Geometry: final body of the model. Coordinates: model frame, mm. A direction names the side the tool comes from. Give positions to 0.01 mm unless a question says otherwise; leave off trailing zeros. Write each loop counter-clockwise with the first axis right and the second up, starting at its lowest first coordinate (ties: lowest second). Pieces come first, ordered by that corner, then holes.
Q1. Line query: line 1 (Y direction, x = 32.35, z = 12.75); line 2 (Y direction, x = 38.5, z = 16.75); line 3 (Y direction, x = -44, z = 17). Output: solid intervals per line, ascending.
Q2. Pin query (flat end, axial travel): pin 1 Ø2 at (x, y) = (-25, 35) entering from -Z; pin 2 Ø2 at (x, y) = (-32.35, 35) entering from +Z; pin 3 Ø6 at (y, z) = (11.5, 6) entering from -X. Return the tip coordinate at first contact, or that it passes through.
Q3. Section A-A (z = 14.5). State how many separate pieces and enclosed holes the cut face has, plus the area to 3 significant figures.
Q4. Mould query, pull axis X, two halves, no side actions, for faces 1 (the cylindrical face through (-41.86, 31.1, 1.97)), 2 (the flat face through (41, 35, 19.5)), 3 (the flat face through (-33, 33, 17.5)). Classes: +X half, -X half, draft (parallel to the pull), parting line (faces both ways), or undercut.
Q5. Reachability of faces 4 (the flat face through (0, -38, 2)), 5 (the flat face through (44.05, 35, 11)), 6 (the flat face through (20.7, -44, 2)) from +Z, -Z, +X, -X, +Y, -Y: full face, straight path, thin tool, end or side. Return the list, or none.
Q6. Section B-B (y = -22.5). Return the cut outline in (x, z).
from build123d import *

# Parameters (mm, degrees)
SKETCH_R        = 1
SKETCH_W        = 23.3
SKETCH_H        = 12.8
SKETCH_W_2      = 76
SKETCH_H_2      = 21
SKETCH_W_3      = 24
SKETCH_H_3      = 16
PAD_DEPTH       = 4
SKETCH005_R     = 1.25
POCKET001_DEPTH = 5
SKETCH002_W     = 23.4
SKETCH002_H     = 6
SKETCH002_W_2   = 3
SKETCH002_H_2   = 30
PAD001_DEPTH    = 13.5
SKETCH008_R     = 1.4
POCKET_DEPTH    = 11
SKETCH007_R     = 1.25
PAD002_DEPTH    = 2
SKETCH004_W     = 19
SKETCH004_H     = 12
POCKET002_DEPTH = 5
SKETCH009_R     = 1.25
POCKET003_DEPTH = 11


with BuildPart() as part:
    # Sketch → Pad (new body)
    with BuildSketch(Plane.XY):
        with BuildLine():
            Line((-11.7, 38), (11.7, 38))
            ThreePointArc((11.7, 38), (13.82132, 38.87868), (14.7, 41))
            Line((14.7, 41), (14.7, 50.8))
            ThreePointArc((17.7, 53.8), (15.57868, 52.92132), (14.7, 50.8))
            Line((17.7, 53.8), (47, 53.8))
            ThreePointArc((50, 50.8), (49.12132, 52.92132), (47, 53.8))
            Line((50, 50.8), (50, 35))
            ThreePointArc((47, 32), (49.12132, 32.87868), (50, 35))
            Line((47, 32), (44, 32))
            ThreePointArc((44, 32), (41.87868, 31.12132), (41, 29))
            Line((41, 29), (41, -29))
            ThreePointArc((41, -29), (41.87868, -31.12132), (44, -32))
            Line((44, -32), (47, -32))
            ThreePointArc((50, -35), (49.12132, -32.87868), (47, -32))
            Line((50, -35), (50, -50.8))
            ThreePointArc((47, -53.8), (49.12132, -52.92132), (50, -50.8))
            Line((47, -53.8), (17.7, -53.8))
            ThreePointArc((14.7, -50.8), (15.57868, -52.92132), (17.7, -53.8))
            Line((14.7, -50.8), (14.7, -41))
            ThreePointArc((14.7, -41), (13.82132, -38.87868), (11.7, -38))
            Line((11.7, -38), (-11.7, -38))
            ThreePointArc((-11.7, -38), (-13.82132, -38.87868), (-14.7, -41))
            Line((-14.7, -41), (-14.7, -50.8))
            ThreePointArc((-17.7, -53.8), (-15.57868, -52.92132), (-14.7, -50.8))
            Line((-17.7, -53.8), (-47, -53.8))
            ThreePointArc((-50, -50.8), (-49.12132, -52.92132), (-47, -53.8))
            Line((-50, -35), (-50, -50.8))
            ThreePointArc((-47, -32), (-49.12132, -32.87868), (-50, -35))
            Line((-47, -32), (-44, -32))
            ThreePointArc((-44, -32), (-41.87868, -31.12132), (-41, -29))
            Line((-41, -29), (-41, 29))
            ThreePointArc((-41, 29), (-41.87868, 31.12132), (-44, 32))
            Line((-44, 32), (-47, 32))
            ThreePointArc((-50, 35), (-49.12132, 32.87868), (-47, 32))
            Line((-50, 50.8), (-50, 35))
            ThreePointArc((-47, 53.8), (-49.12132, 52.92132), (-50, 50.8))
            Line((-47, 53.8), (-17.7, 53.8))
            ThreePointArc((-14.7, 50.8), (-15.57868, 52.92132), (-17.7, 53.8))
            Line((-14.7, 50.8), (-14.7, 41))
            ThreePointArc((-14.7, 41), (-13.82132, 38.87868), (-11.7, 38))
        make_face()
        with Locations((-46.5, 44.4)):
            Circle(SKETCH_R, mode=Mode.SUBTRACT)
        with Locations((-18.2, 44.4)):
            Circle(SKETCH_R, mode=Mode.SUBTRACT)
        with Locations((18.2, 44.4)):
            Circle(SKETCH_R, mode=Mode.SUBTRACT)
        with Locations((46.5, 44.4)):
            Circle(SKETCH_R, mode=Mode.SUBTRACT)
        with Locations((-46.5, -44.4)):
            Circle(SKETCH_R, mode=Mode.SUBTRACT)
        with Locations((-18.2, -44.4)):
            Circle(SKETCH_R, mode=Mode.SUBTRACT)
        with Locations((18.2, -44.4)):
            Circle(SKETCH_R, mode=Mode.SUBTRACT)
        with Locations((46.5, -44.4)):
            Circle(SKETCH_R, mode=Mode.SUBTRACT)
        with Locations((-32.35, 44.4)):
            Rectangle(SKETCH_W, SKETCH_H, mode=Mode.SUBTRACT)
        with Locations((32.35, 44.4)):
            Rectangle(SKETCH_W, SKETCH_H, mode=Mode.SUBTRACT)
        with Locations((32.35, -44.4)):
            Rectangle(SKETCH_W, SKETCH_H, mode=Mode.SUBTRACT)
        with Locations((-32.35, -44.4)):
            Rectangle(SKETCH_W, SKETCH_H, mode=Mode.SUBTRACT)
        with Locations((0, 21.5)):
            Rectangle(SKETCH_W_2, SKETCH_H_2, mode=Mode.SUBTRACT)
        with Locations((0, -21.5)):
            Rectangle(SKETCH_W_2, SKETCH_H_2, mode=Mode.SUBTRACT)
        with Locations((26, 0)):
            Rectangle(SKETCH_W_3, SKETCH_H_3, mode=Mode.SUBTRACT)
        with BuildLine():
            Line((-38, 8), (-38, -8))
            Line((-38, -8), (-14, -8))
            Line((-14, -8), (-14, 8))
            Line((-14, 8), (-25.04196, 8))
            ThreePointArc((-30.95804, 8), (-28, 5.5), (-25.04196, 8))
            Line((-30.95804, 8), (-38, 8))
        make_face(mode=Mode.SUBTRACT)
        with BuildLine():
            ThreePointArc((5.95804, -8), (3, -5.5), (0.04196, -8))
            Line((-11, -8), (0.04196, -8))
            Line((-11, 8), (-11, -8))
            Line((11, 8), (-11, 8))
            Line((11, -8), (11, 8))
            Line((5.95804, -8), (11, -8))
        make_face(mode=Mode.SUBTRACT)
    extrude(amount=PAD_DEPTH)

    # Sketch005 → Pocket001 (cut)
    with BuildSketch(Plane.XY.offset(4)):
        with Locations((3, -8.5)):
            Circle(SKETCH005_R)
        with Locations((-28, 8.5)):
            Circle(SKETCH005_R)
    extrude(amount=-POCKET001_DEPTH, mode=Mode.SUBTRACT)

    # Sketch002 (on Face5 of Pocket001) → Pad001 (join)
    with BuildSketch(Plane.XY.offset(4)):
        with Locations((-32.35, 35)):
            Rectangle(SKETCH002_W, SKETCH002_H)
        with Locations((32.35, 35)):
            Rectangle(SKETCH002_W, SKETCH002_H)
        with Locations((-32.35, -35)):
            Rectangle(SKETCH002_W, SKETCH002_H)
        with Locations((32.35, -35)):
            Rectangle(SKETCH002_W, SKETCH002_H)
        with Locations((39.5, 0)):
            Rectangle(SKETCH002_W_2, SKETCH002_H_2)
    extrude(amount=PAD001_DEPTH)

    # Sketch008 → Pocket (cut)
    with BuildSketch(Plane.XY.offset(17.5)):
        with Locations((-32.35, 35)):
            Circle(SKETCH008_R)
        with Locations((32.35, 35)):
            Circle(SKETCH008_R)
        with Locations((-32.35, -35)):
            Circle(SKETCH008_R)
        with Locations((32.35, -35)):
            Circle(SKETCH008_R)
    extrude(amount=-POCKET_DEPTH, mode=Mode.SUBTRACT)

    # Sketch007 (on Face112 of Pocket) → Pad002 (join)
    with BuildSketch(Plane.XY.offset(17.5)):
        with Locations((-40.85, 35)):
            Circle(SKETCH007_R)
        with Locations((-23.85, 35)):
            Circle(SKETCH007_R)
        with Locations((23.85, 35)):
            Circle(SKETCH007_R)
        with Locations((40.85, 35)):
            Circle(SKETCH007_R)
        with Locations((-40.85, -35)):
            Circle(SKETCH007_R)
        with Locations((-23.85, -35)):
            Circle(SKETCH007_R)
        with Locations((23.85, -35)):
            Circle(SKETCH007_R)
        with Locations((40.85, -35)):
            Circle(SKETCH007_R)
    extrude(amount=PAD002_DEPTH)

    # Sketch004 (on Face105 of Pad002) → Pocket002 (cut)
    with BuildSketch(Plane.YZ.offset(41)):
        with Locations((0, 10.07)):
            Rectangle(SKETCH004_W, SKETCH004_H)
    extrude(amount=-POCKET002_DEPTH, mode=Mode.SUBTRACT)

    # Sketch009 (on Face4 of Pocket002) → Pocket003 (cut)
    with BuildSketch(Plane(origin=(0, 0, 0), x_dir=(1, 0, 0), z_dir=(0, 0, -1))):
        with Locations((28, 35)):
            Circle(SKETCH009_R)
        with Locations((-25, 35)):
            Circle(SKETCH009_R)
        with Locations((-25, -35)):
            Circle(SKETCH009_R)
        with Locations((28, -35)):
            Circle(SKETCH009_R)
    extrude(amount=-POCKET003_DEPTH, mode=Mode.SUBTRACT)


solid = part.part
Computed:
1. line 1: y = -38 to -36.4, -33.6 to -32, 32 to 33.6, 36.4 to 38
1. line 2: y = -38 to -32, -15 to 15, 32 to 38
1. line 3: y = -38 to -32, 32 to 38
2. pin 1: stops at z = 11
2. pin 2: stops at z = 6.5
2. pin 3: stops at x = -41
3. separate pieces: 6
3. enclosed holes: 4
3. area: 570 mm2
4. face 1: -X half
4. face 2: draft
4. face 3: undercut
5. face 4: +Z, -Z, -Y
5. face 5: +Z, +X, +Y, -Y
5. face 6: +Z, -Z
6. outline: (-41, 0) - (-38, 0) - (-38, 4) - (-41, 4) - close; (38, 0) - (41, 0) - (41, 4) - (38, 4) - close
